Check sheet for the modelled part. Datum: model origin and axes. Units: mm. A direction names the side the tool comes from. Coordinates: 2 decimals unless noted, no trailing zeros. Loops run counter-clockwise (first coordinate to the right, second up) from the corner with the lowest first, then second, coordinate; pieces in that order, holes last. Notation, with made-up numbers: M -21,-12.75 L 37,-12.75 A7 ccw 37,-3.75 Z; hole C 9,9 d11. An arc over 180 degrees is marked long. Return JSON: item names as keys, results as strings.
from build123d import *

# Parameters (mm, degrees)
F0_W     = 101.6
F0_H     = 95.25
F0_R     = 2.3114
F1_DEPTH = 8.255
F2_R     = 5.08
F3_W     = 101.6
F3_H     = 29.464
F4_DEPTH = 8.382


# Not quite as in the source:
# - a feature names something its author has since deleted; it is built from what else it names


with BuildPart() as f1:
    # F0 (on Top) → F1 (new body)
    with BuildSketch(Plane.XY):
        Rectangle(F0_W, F0_H)
        Polygon((38.1, -15.24), (0, -15.24), (-38.1, -15.24), (-38.1, 15.24), (-25.4, 15.24), (0, 15.24), (25.4, 15.24), (38.1, 15.24), align=None, mode=Mode.SUBTRACT)
        Polygon((-38.1, -15.24), (0, -15.24), (38.1, -15.24), (38.1, 15.24), (25.4, 15.24), (0, 15.24), (-25.4, 15.24), (-38.1, 15.24), align=None)
        with Locations((-31.75, -7.6708)):
            Circle(F0_R, mode=Mode.SUBTRACT)
        with Locations((31.75, -7.6708)):
            Circle(F0_R, mode=Mode.SUBTRACT)
        with Locations((-31.75, 5.0292)):
            Circle(F0_R, mode=Mode.SUBTRACT)
        with Locations((31.75, 5.0292)):
            Circle(F0_R, mode=Mode.SUBTRACT)
    extrude(amount=F1_DEPTH)

    # F2
    f2_edges = [f1.edges().sort_by_distance(p)[0] for p in [
        (-50.8, 47.625, 4.1275),
        (50.8, 47.625, 4.1275),
        (50.8, -47.625, 4.1275),
        (-50.8, -47.625, 4.1275),
    ]]
    fillet(f2_edges, radius=F2_R)

    # F3 (on face) → F4 (join)
    with BuildSketch(Plane(origin=(0, 0, 0), x_dir=(1, 0, 0), z_dir=(0, 0, -1))):
        with Locations((0, 27.813)):
            Rectangle(F3_W, F3_H)
        with Locations((0, -27.813)):
            Rectangle(F3_W, F3_H)
    extrude(amount=F4_DEPTH)


solid = f1.part
1) Section check A-A on x = -31.75. Record the cut outline in (y, z) (3 decimals), then the cut area to 3 significant figures.
Answers:
{"outline": "M -47.625,0 L -42.545,0 L -42.545,-8.382 L -13.081,-8.382 L -13.081,0 L -9.982,0 L -9.982,8.255 L -47.625,8.255 Z; M -5.359,0 L 2.718,0 L 2.718,8.255 L -5.359,8.255 Z; M 7.341,0 L 13.081,0 L 13.081,-8.382 L 42.545,-8.382 L 42.545,0 L 47.625,0 L 47.625,8.255 L 7.341,8.255 Z", "area": "1,200 mm²"}
2) Go/stop test with flat-tipped pins: pin 1 Ø3.5 at (x, y) = (31.75, 5.03) entering from -Z; pin 2 Ø4 at (x, y) = (21, -45.5) entering from -Z; pin 3 Ø9 at (x, z) = (21.5, -3) entering from -Y (3 decimals); pin 4 Ø2.5 at (x, z) = (6, -5.5) entering from +Y (3 decimals). Record where each tip stops, or that it passes through.
Answers:
{"pin 1": "through", "pin 2": "z = 0", "pin 3": "y = -47.625", "pin 4": "y = 42.545"}
3) Draft check along X on faces 1 (the face through (-49.35, -46.1, 4.19)), 2 (the face through (33.955, -6.977, 4.07)), 3 (the face through (-1, 47.625, 4)). Enter one of: +X half, -X half, draft (parallel to the pull), parting line (faces both ways), or undercut.
Answers:
{"face 1": "-X half", "face 2": "undercut", "face 3": "draft"}
4) Section check B-B on x = 19.5. Record the cut outline in (y, z) (3 decimals).
Answers:
{"outline": "M -47.625,0 L -42.545,0 L -42.545,-8.382 L -13.081,-8.382 L -13.081,0 L 13.081,0 L 13.081,-8.382 L 42.545,-8.382 L 42.545,0 L 47.625,0 L 47.625,8.255 L -47.625,8.255 Z"}
5) Section check C-C on y = 1. Record the cut outline in (x, z) (3 decimals).
Answers:
{"outline": "M -50.8,0 L 50.8,0 L 50.8,8.255 L -50.8,8.255 Z"}
6) Scan lines: line 1 along Y through (x, z) = (31.75, 2) (3 decimals); line 2 along X through (y, z) = (5, 5.75); line 3 along Y through (x, z) = (-33.5, -6.25) (3 decimals). Record each from-to range of solid material in increasing order. Write a range as [from, to].
Answers:
{"line 1": "[-47.625, -9.982], [-5.359, 2.718], [7.341, 47.625]", "line 2": "[-50.8, -34.06], [-29.44, 29.44], [34.06, 50.8]", "line 3": "[-42.545, -13.081], [13.081, 42.545]"}
7) Set-up check for faces 4 (the face through (-1, 13.081, -4)), 5 (the face through (-1, 45, 0)), 6 (the face through (-33.454, 6.591, 4.07)), 7 (the face through (-49.35, 46.1, 4.19)), 8 (the face through (-1, -45, 0)): record each of +Z, -Z, +X, -X, +Y, -Y from which the full face is reachable in a straight line by a thin tool's end or side.
Answers:
{"face 4": "-Z, +X, -X", "face 5": "-Z, +X, -X, +Y", "face 6": "+Z, -Z", "face 7": "+Z, -Z, -X, +Y", "face 8": "-Z, +X, -X, -Y"}
